Here's the drawing with two shaded views (mm, measured from the low corner). I have some questions. Give positions to 0.01 mm unless a question says otherwise; leave off trailing zeros. Loops run counter-clockwise (first coordinate to the right, second up) from the corner with the lowest first, then second, coordinate; pieces in that order, holes last. Notation, with made-up numbers: (-32, -18) -> (10, -18) arc R9 cw to (10, -4) -> close; hole circle Ø10 at (-6, 16). An arc over 180 degrees is marked (long way). Write each question's results on one line, items separated by ' | '. Start each with the question number.
Q1. If we section it at C-C, the plane y = 4.3: Give the number of separate pieces and of enclosed holes in the cut face.
Q2. If we section it at A-A, the plane x = 27.5: List the corners of the cut face in (y, z) for me, plus the area to 3 significant figures.
Q3. If I drill on line 1 along Z through (x, y) = (19.75, 4.75) (1 decimal); line 2 along X through (y, z) = (3.4, 24); line 3 along X through (y, z) = (4.75, 82.5) (1 decimal), over which ranges is the centre line in solid material (lowest first)?
Q4. If we section it at B-B, the plane z = 89.5: List the corners of the cut face in (x, y) for me, plus the area to 3 significant figures.
Q5. If we section it at D-D, the plane x = 60.5: List the corners of the cut face in (y, z) for me.
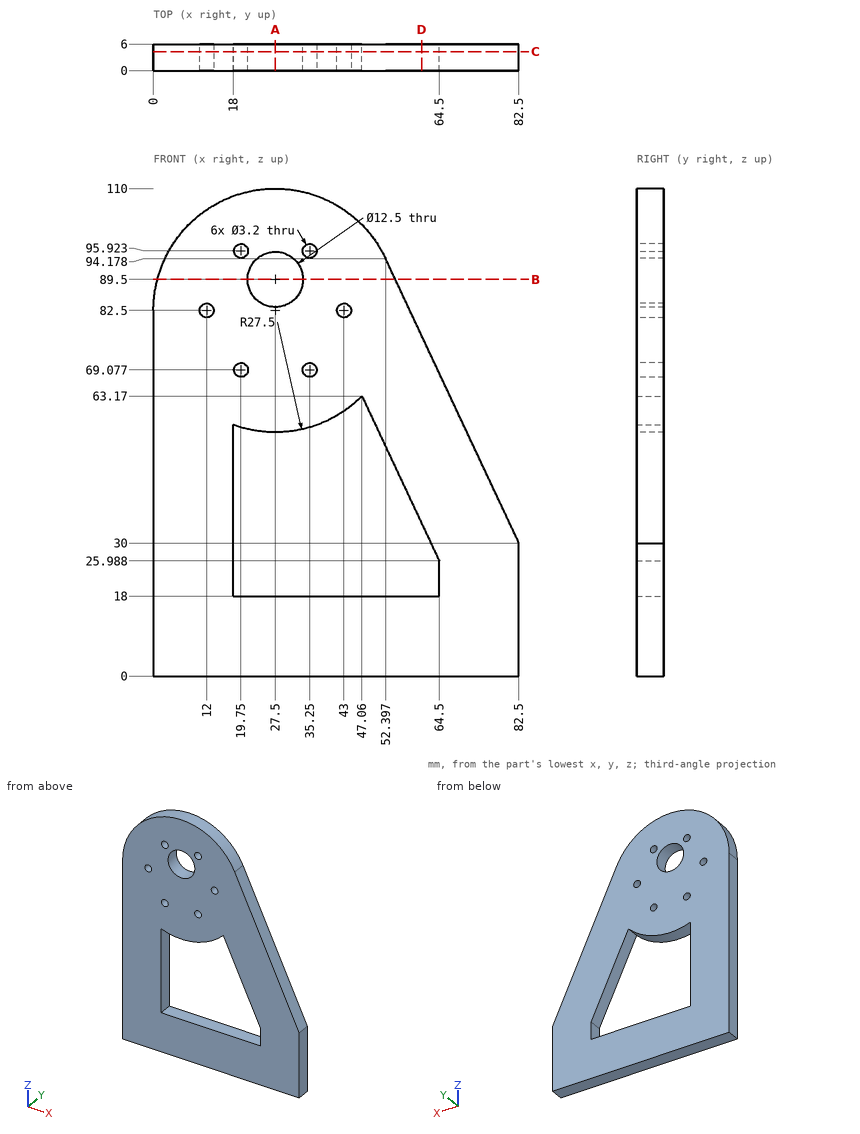
Final values:
1) separate pieces: 1 | enclosed holes: 8
2) outline: (0, 0) -> (6, 0) -> (6, 18) -> (0, 18) -> close; (0, 55) -> (6, 55) -> (6, 83.25) -> (0, 83.25) -> close; (0, 95.75) -> (6, 95.75) -> (6, 110) -> (0, 110) -> close | area: 363 mm²
3) line 1: z = 0 to 18, 56.1 to 67.5, 70.7 to 94.3, 97.5 to 108.9 | line 2: x = 0 to 18, 64.5 to 82.5 | line 3: x = 0 to 10.4, 13.6 to 41.4, 44.6 to 57.9
4) outline: (0.91, 0) -> (21.25, 0) -> (21.25, 6) -> (0.91, 6) -> close; (33.75, 0) -> (54.59, 0) -> (54.59, 6) -> (33.75, 6) -> close | area: 247 mm²
5) outline: (0, 0) -> (6, 0) -> (6, 18) -> (0, 18) -> close; (0, 34.52) -> (6, 34.52) -> (6, 76.9) -> (0, 76.9) -> close
